Build history of the part. All positions in model axes, mm. A direction names the side the tool comes from. Give positions to 0.01 mm unless a question says otherwise; leave off trailing zeros. Loops run counter-clockwise (first coordinate to the right, second up) from the corner with the lowest first, then second, coordinate; pieces in that order, holes last.
1) Band-saw the part on D-D on x = 68. List the corners of the cut face in (y, z).
2) Band-saw the part on A-A on z = 185. List the corners of the cut face in (x, y).
3) Flat gauge pins, fed straight in: P1, Ø1.7, axis at x = 37, z = 2.5, coming from the -Y side; P2, Ø8, axis at y = 55.5, z = 111.5, coming from the +X side; P3, Ø13, axis at x = -112, z = 248.5, coming from the -Y side; P4, Ø3, axis at y = 30, z = 300, coming from the -X side. Where does each tip first touch, or does it go through?
4) Wall check: line 1 (Z direction, x = 223, y = 99); line 2 (Y direction, x = -74, z = 314); line 3 (Y direction, x = 127, z = 209). Give the ranges that are in metal, low to high.
5) Band-saw the part on C-C on z = 62. List the corners of the cut face in (x, y).
6) Band-saw the part on B-B on x = -58.5. List the corners of the cut face in (y, z).
7) 3-axis set-ups, long thin cutter, end or side, ignore diameter. For faces 1 (the flat face through (183, 37, 6)), 2 (the flat face through (287.123, 37.547, 294.47)), 3 (the flat face through (-51, 8.001, 169)): which of +Z, -Z, +X, -X, +Y, -Y reach the whole face in a straight line?
8) Two-plate mould, pull along Y, no slides. Class faces 4 (the flat face through (-123, 26.001, 169)), 5 (the flat face through (38, 37, 6)), 6 (the flat face through (-99.248, 16, 169)): +Y half, -Y half, draft (parallel to the pull), parting line (faces both ways), or undercut.
Autodesk Inventor part; units mm, degrees
ref_plane "YZ Plane" through (0, 0, 0) normal (1, 0, 0) x (0, 1, 0)
ref_plane "XZ Plane" through (0, 0, 0) normal (0, 1, 0) x (-1, 0, 0)
ref_plane "XY Plane" through (0, 0, 0) normal (0, 0, 1) x (1, 0, 0)
sketch "Sketch1" plane through (0, 0, 0) normal (0, 0, 1) x (1, 0, 0)
  line L0 (0, 0) -> (220, 0)
  line L1 (110, 0) -> (110, 266.5) construction
  line L2 (110, 266.5) -> (317.5, 266.5)
  line L3 (110, 266.5) -> (-97.5, 266.5)
  line L4 (220, 0) -> (340, 0) construction
  line L5 (317.5, 266.5) -> (350.6537, 14.673)
  line L6 (317.5, 266.5) -> (571.5, 266.5) construction
  line L7 (350.6537, 14.673) -> (220, 0)
  line L8 (-97.5, 266.5) -> (-144.2482, 26.0013)
  line L9 (-97.5, 266.5) -> (147.5, 266.5) construction
  line L10 (-144.2482, 26.0013) -> (-101.2482, 26.0013)
  line L11 (-99.2482, 24.0013) -> (-99.2482, 8.0013)
  line L12 (-99.2482, 8.0013) -> (-2, 8.0013)
  line L13 (0, 6.0013) -> (0, 0)
  arc A0 (0, 6.0013) -> (-2, 8.0013) centre (-2, 6.0013) ccw
  arc A1 (-99.2482, 24.0013) -> (-101.2482, 26.0013) centre (-101.2482, 24.0013) ccw
  point P0 (-99.2482, 26.0013)
  dimension "d0" = 220
  dimension "d1" = 266.5
  dimension "d7" = 254
  dimension "d8" = 82.5
  dimension "d9" = 245
  dimension "d10" = 101
  dimension "d11" = 45
  dimension "d12" = 18
  dimension "d14" = 415
  dimension "d15" = 2
  dimension "d16" = 2
extrude "Extrusion1" add sketch "Sketch1" along normal blind 342
sketch "Sketch3" plane through (317.5, 266.5, 342) normal (0.9914, 0.1305, 0) x (0, 0, -1)
  circle A0 centre (182, -91.5) radius 70
  line L0 (342, -254) -> (342, 0)
  line L1 (342, 0) -> (0, 0)
  line L2 (252, -91.5) -> (342, -91.5) construction
  line L3 (182, -21.5) -> (182, 0) construction
  point P0 (342, -222.778)
  dimension "d22" = 140
  dimension "d26" = 160
  dimension "d27" = 70
  dimension "d28" = 91.5
  dimension "d29" = 70
extrude "Extrusion2" cut sketch "Sketch3" against normal blind 10
sketch "Sketch4" plane through (317.5, 266.5, 342) normal (0.9914, 0.1305, 0) x (0, 0, -1)
  line L0 (342, 0) -> (0, 0)
  line L1 (0, -254) -> (0, 0)
  circle A0 centre (51, -45) radius 15
  line L2 (51, 0) -> (51, -45) construction
  line L3 (51, -45) -> (0, -45) construction
  circle A1 centre (47.75, -223.25) radius 15.75
  line L4 (342, -254) -> (0, -254)
  line L5 (47.75, -223.25) -> (0, -223.25) construction
  line L6 (47.75, -223.25) -> (47.75, -254) construction
  point P0 (342, -222.778)
  dimension "d34" = 30
  dimension "d37" = 45
  dimension "d38" = 51
  dimension "d39" = 31.5
  dimension "d42" = 30.75
  dimension "d43" = 47.75
extrude "Extrusion3" cut sketch "Sketch4" against normal blind 60
sketch "Sketch5" plane through (0, 0, 0) normal (0, 0, -1) x (-1, 0, 0)
  line L0 (-350.6537, 14.673) -> (-317.5, 266.5)
  line L1 (-317.5, 266.5) -> (97.5, 266.5)
  circle A0 centre (-142.0425, 167.4324) radius 80.5
  line L2 (-142.0425, 247.9324) -> (-142.0425, 266.9324) construction
  line L3 (-142.0425, 167.4324) -> (-330.5425, 167.4324) construction
  point P0 (0, 0)
  dimension "d49" = 161
  dimension "d50" = 19
  dimension "d52" = 188.5
extrude "Extrusion4" add sketch "Sketch5" along normal blind 26
sketch "Sketch6" plane through (142.0425, 167.4324, -26) normal (0, 0, -1) x (-1, 0, 0)
  circle A0 centre (0, 0) radius 29
  point P0 (142.0425, -167.4324)
  dimension "d55" = 58
extrude "Extrusion5" cut sketch "Sketch6" against normal through all
sketch "Sketch7" plane through (0, 0, 0) normal (0, 0, -1) x (-1, 0, 0)
  line L0 (-39.1667, 56.5) -> (-35.7652, 56.5)
  line L1 (-45.3265, 16.5) -> (-29.6054, 16.5)
  line L2 (-48.9954, 48.3429) -> (-53.1895, 25.9743)
  line L3 (-25.9365, 48.3429) -> (-21.7424, 25.9743)
  arc A0 (-39.1667, 56.5) -> (-48.9954, 48.3429) centre (-39.1667, 46.5) ccw
  arc A1 (-25.9365, 48.3429) -> (-35.7652, 56.5) centre (-35.7652, 46.5) ccw
  arc A2 (-53.1895, 25.9743) -> (-45.3265, 16.5) centre (-45.3265, 24.5) ccw
  arc A3 (-29.6054, 16.5) -> (-21.7424, 25.9743) centre (-29.6054, 24.5) ccw
  line L4 (0, 0) -> (-220, 0)
  line L5 (-110, 0) -> (-110, 69.6289)
  line L6 (-180.8333, 56.5) -> (-184.2348, 56.5)
  line L7 (-174.6735, 16.5) -> (-190.3946, 16.5)
  line L8 (-171.0046, 48.3429) -> (-166.8105, 25.9743)
  line L9 (-194.0635, 48.3429) -> (-198.2576, 25.9743)
  arc A4 (-171.0046, 48.3429) -> (-180.8333, 56.5) centre (-180.8333, 46.5) ccw
  arc A5 (-184.2348, 56.5) -> (-194.0635, 48.3429) centre (-184.2348, 46.5) ccw
  arc A6 (-174.6735, 16.5) -> (-166.8105, 25.9743) centre (-174.6735, 24.5) ccw
  arc A7 (-198.2576, 25.9743) -> (-190.3946, 16.5) centre (-190.3946, 24.5) ccw
  point P0 (-47.466, 56.5)
  point P1 (-27.466, 56.5)
  point P2 (-54.966, 16.5)
  point P3 (-19.966, 16.5)
  point P4 (-172.534, 56.5)
  point P5 (-192.534, 56.5)
  point P6 (-165.034, 16.5)
  point P7 (-200.034, 16.5)
  dimension "d69" = 20
  dimension "d70" = 35
  dimension "d72" = 10
  dimension "d73" = 8
extrude "Extrusion6" cut sketch "Sketch7" against normal blind 6
fillet "Fillet1" radius 2 8 edges at (182.534, 56.5, 6) (174.447, 54.1951, 6) (168.9075, 37.1586, 6) (168.5174, 19.3909, 6) (182.534, 16.5, 6) (196.5507, 19.3909, 6) (196.1606, 37.1586, 6) (190.6211, 54.1951, 6)
fillet "Fillet2" radius 2 8 edges at (51.0925, 37.1586, 6) (45.553, 54.1951, 6) (37.466, 56.5, 6) (29.3789, 54.1951, 6) (23.8394, 37.1586, 6) (23.4493, 19.3909, 6) (37.466, 16.5, 6) (51.4826, 19.3909, 6)
ref_plane "Work Plane2" through (142.0425, 167.4324, -26) normal (-1, 0, 0) x (0, 0, 1)
properties part number "Gearbox"
Findings below:
1. outline: (0, 0) - (135.84, 0) - (135.84, -26) - (199.02, -26) - (199.02, 0) - (266.5, 0) - (266.5, 342) - (0, 342) - close
2. outline: (-144.25, 26) - (-101.25, 26) arc R2 cw to (-99.25, 24) - (-99.25, 8) - (-2, 8) arc R2 cw to (0, 6) - (0, 0) - (220, 0) - (350.65, 14.67) - (337.98, 110.96) - (328.06, 109.65) - (310.99, 239.3) - (320.91, 240.61) - (317.5, 266.5) - (-97.5, 266.5) - close; hole circle Ø58 at (142.04, 167.43)
3. P1: stops at y = 0
3. P2: stops at x = 345.81
3. P3: stops at y = 26
3. P4: stops at x = -143.76
4. line 1: z = 0 to 342
4. line 2: y = 8 to 266.5
4. line 3: y = 0 to 142.64, 192.23 to 266.5
5. outline: (-144.25, 26) - (-101.25, 26) arc R2 cw to (-99.25, 24) - (-99.25, 8) - (-2, 8) arc R2 cw to (0, 6) - (0, 0) - (220, 0) - (350.65, 14.67) - (317.5, 266.5) - (-97.5, 266.5) - close; hole circle Ø58 at (142.04, 167.43)
6. outline: (8, 0) - (266.5, 0) - (266.5, 342) - (8, 342) - close
7. face 1: -Z
7. face 2: none
7. face 3: +Z, -Z, -X, -Y
8. face 4: -Y half
8. face 5: undercut
8. face 6: draft
